from build123d import *

# Parameters (mm, degrees)
F1_DEPTH = 2
F2_W     = 2
F2_H     = 2
F3_DEPTH = 5
F5_DEPTH = 2


with BuildPart() as f1:
    # F0 (on Right) → F1 (new body)
    with BuildSketch(Plane.YZ):
        with BuildLine():
            ThreePointArc((9.219544, 5), (8.742813, 5.120951), (8.381404, 5.454545))
            ThreePointArc((8.381404, 5.454545), (-10, 0), (8.381404, -5.454545))
            ThreePointArc((8.381404, -5.454545), (8.742813, -5.120951), (9.219544, -5))
            Line((9.219544, -5), (13.660254, -5))
            ThreePointArc((13.660254, -5), (14.367361, -5.292893), (14.660254, -6))
            Line((14.660254, -6), (14.660254, -30.115784))
            Line((14.660254, -30.115784), (16.660254, -30.115784))
            Line((16.660254, -30.115784), (16.660254, -6))
            ThreePointArc((16.660254, -6), (15.781575, -3.878679), (13.660254, -3))
            Line((13.660254, -3), (9.219544, -3))
            ThreePointArc((9.219544, -3), (7.78935, -3.362852), (6.705123, -4.363636))
            ThreePointArc((6.705123, -4.363636), (-8, 0), (6.705123, 4.363636))
            ThreePointArc((6.705123, 4.363636), (7.78935, 3.362852), (9.219544, 3))
            Line((9.219544, 3), (11.660254, 3))
            Line((11.660254, 3), (11.660254, 5))
            Line((11.660254, 5), (9.219544, 5))
        make_face()
    extrude(amount=F1_DEPTH)

    # F2 (on face) → F3 (join)
    with BuildSketch(Plane.YZ.offset(2)):
        with Locations((10.660254, 4)):
            Rectangle(F2_W, F2_H)
    extrude(amount=F3_DEPTH)

    # F4 (on face) → F5 (join)
    with BuildSketch(Plane.YZ.offset(7)):
        with BuildLine():
            ThreePointArc((9.219544, 5), (8.742813, 5.120951), (8.381404, 5.454545))
            ThreePointArc((8.381404, 5.454545), (-10, 0), (8.381404, -5.454545))
            ThreePointArc((8.381404, -5.454545), (8.742813, -5.120951), (9.219544, -5))
            Line((9.219544, -5), (12.623615, -5))
            ThreePointArc((12.623615, -5), (13.330721, -5.292893), (13.623615, -6))
            Line((13.623615, -6), (13.623615, -23.685562))
            Line((13.623615, -23.685562), (15.623615, -23.685562))
            Line((15.623615, -23.685562), (15.623615, -6))
            ThreePointArc((15.623615, -6), (14.744935, -3.878679), (12.623615, -3))
            Line((12.623615, -3), (9.219544, -3))
            ThreePointArc((9.219544, -3), (7.78935, -3.362852), (6.705123, -4.363636))
            ThreePointArc((6.705123, -4.363636), (-8, 0), (6.705123, 4.363636))
            ThreePointArc((6.705123, 4.363636), (7.78935, 3.362852), (9.219544, 3))
            Line((9.219544, 3), (11.660254, 3))
            Line((11.660254, 3), (11.660254, 5))
            Line((11.660254, 5), (9.219544, 5))
        make_face()
    extrude(amount=F5_DEPTH)


solid = f1.part
Geometry check sheet. Reference: the model listing, model coordinates, mm. A direction names the side the tool comes from. Give positions to 0.01 mm unless a question says otherwise; leave off trailing zeros. Write each loop counter-clockwise with the first axis right and the second up, starting at its lowest first coordinate (ties: lowest second). Pieces come first, ordered by that corner, then holes. Notation, with made-up numbers: M 26,-30.5 L 67,-30.5 A9 ccw 67,-13.5 Z; hole C 76.25,3 d11. An arc over 180 degrees is marked long. One line per question, with ' | ' between items.
1. Gauge pin test, flat ends, axial feed: pin 1 (0.6 mm diameter, centred on x = 0.5, y = 12, fed in from +Z); pin 2 (2 mm diameter, centred on x = 3, y = 10, fed in from +Z); pin 3 (2 mm diameter, centred on x = 1.5, z = -14.5, fed in from -Y). Record the tip position at first contact, or that the pin passes through.
Ans:
pin 1: z = -3 | pin 2: z = 5 | pin 3: y = 14.66
2. Cross-section at D-D (z = -9). Enter the section's corners in (x, y).
Ans:
outline: M 0,-4.36 L 2,-4.36 L 2,4.36 L 0,4.36 Z; M 0,14.66 L 2,14.66 L 2,16.66 L 0,16.66 Z; M 7,-4.36 L 9,-4.36 L 9,4.36 L 7,4.36 Z; M 7,13.62 L 9,13.62 L 9,15.62 L 7,15.62 Z
3. Cross-section at C-C (x = 1). Enter the section's corners in (y, z).
Ans:
outline: M 6.71,-4.36 A8 cw long 6.71,4.36 A3 ccw 9.22,3 L 11.66,3 L 11.66,5 L 9.22,5 A1 cw 8.38,5.45 A10 ccw long 8.38,-5.45 A1 cw 9.22,-5 L 13.66,-5 A1 cw 14.66,-6 L 14.66,-30.12 L 16.66,-30.12 L 16.66,-6 A3 ccw 13.66,-3 L 9.22,-3 A3 ccw Z
4. Cross-section at B-B (z = -15.5). Enter the section's corners in (x, y), plus the area to 3 significant figures.
Ans:
outline: M 0,14.66 L 2,14.66 L 2,16.66 L 0,16.66 Z; M 7,13.62 L 9,13.62 L 9,15.62 L 7,15.62 Z | area: 8.00 mm2
5. Mould release check, pull along X, two halves, no side actions. Record for faces 5 (the face through (7.986, 8.737, -5.124)), 6 (the face through (7, 5, -7)), 7 (the face through (9, 7, -6)): released by +X, released by -X, zero draft, split by the parting line, or undercut.
Ans:
face 5: zero draft | face 6: undercut | face 7: released by +X
6. Scan lines: line 1 along Z through (x, y) = (7.6, 0); line 2 along Z through (x, y) = (1, 11.25); line 3 along X through (y, z) = (7.5, -6). Record each from-to range of solid material in increasing order. Write a range as from..to.
Ans:
line 1: -10..-8, 8..10 | line 2: -5..-3, 3..5 | line 3: 0..2, 7..9
7. Set-up check for faces 1 (the face through (8, 13.624, -15)), 2 (the face through (0.99, 7.81, -3.35)), 3 (the face through (8, 15, -23.686)), 4 (the face through (4, 10, 5)): record each of +Z, -Z, +X, -X, +Y, -Y from which the full face is reachable in a straight line by a thin tool's end or side.
Ans:
face 1: -Z, +X, -X | face 2: +X, -X | face 3: -Z, +X, +Y, -Y | face 4: +Z, +X, -X, +Y
8. Cross-section at A-A (y = 0). Enter the section's corners in (x, z).
Ans:
outline: M 0,-10 L 2,-10 L 2,-8 L 0,-8 Z; M 0,8 L 2,8 L 2,10 L 0,10 Z; M 7,-10 L 9,-10 L 9,-8 L 7,-8 Z; M 7,8 L 9,8 L 9,10 L 7,10 Z
